```python
from build123d import *

# Parameters (mm, degrees)
SKETCH_1_R          = 1.6
SKETCH_1_R_2        = 29
SKETCH_1_R_3        = 1.1
EXTRUDE_1_DEPTH     = 2
FILLET_1_R          = 15
FILLET_2_R          = 10
FILLET_3_R          = 2
SKETCH_2_R          = 1.6
CUT_EXTRUDE_1_DEPTH = 124.188027016
CUT_EXTRUDE_2_DEPTH = 124.188027016
CUT_EXTRUDE_3_DEPTH = 124.188027016
FILLET_4_R          = 10


with BuildPart() as part:
    # 草图1 → 凸台-拉伸1 (new body)
    with BuildSketch(Plane.XY):
        with BuildLine():
            Line((0, 34), (0, 60))
            Line((0, 60), (-75, 60))
            Line((-75, 60), (-104.5, 42))
            Line((-104.5, 42), (-104.5, 10))
            Line((-104.5, 10), (-91.5, 10))
            Line((-91.5, 10), (-91.5, 0))
            Line((-91.5, 0), (-73.5, 0))
            Line((-73.5, 0), (-73.5, 6))
            Line((-73.5, 6), (-60.5, 6))
            Line((-60.5, 6), (-60.5, 0))
            Line((-60.5, 0), (-33, 0))
            Line((-33, 0), (-33, 6))
            Line((-33, 6), (-20, 6))
            Line((-20, 6), (-20, 0))
            Line((-20, 0), (0, 0))
            Line((0, 0), (5, 0))
            Line((5, 0), (8.183105221, -31.876446495))
            ThreePointArc((8.183105221, -31.876446495), (46.840501722, -65.154195343), (82, -28.2))
            Line((82, -28.2), (82, -2))
            Line((82, -2), (50, 34))
            Line((50, 34), (0, 34))
        make_face()
        with Locations((-86.5, 5)):
            Circle(SKETCH_1_R, mode=Mode.SUBTRACT)
        with Locations((-5, 5)):
            Circle(SKETCH_1_R, mode=Mode.SUBTRACT)
        with Locations((45, -28.2)):
            Circle(SKETCH_1_R_2, mode=Mode.SUBTRACT)
        with Locations((-35, 57)):
            Circle(SKETCH_1_R, mode=Mode.SUBTRACT)
        with Locations((-55, 57)):
            Circle(SKETCH_1_R, mode=Mode.SUBTRACT)
        with Locations((-87.5, 46.515606374)):
            Circle(SKETCH_1_R, mode=Mode.SUBTRACT)
        with Locations((-15.4, 48.1)):
            Circle(SKETCH_1_R_3, mode=Mode.SUBTRACT)
        with Locations((-15.4, 30.1)):
            Circle(SKETCH_1_R_3, mode=Mode.SUBTRACT)
        with Locations((-60.6, 48.1)):
            Circle(SKETCH_1_R_3, mode=Mode.SUBTRACT)
        with Locations((-60.6, 30.1)):
            Circle(SKETCH_1_R_3, mode=Mode.SUBTRACT)
        with Locations((-5, 55)):
            Circle(SKETCH_1_R, mode=Mode.SUBTRACT)
    extrude(amount=EXTRUDE_1_DEPTH)

    # 圆角1
    fillet_1_edges = [part.edges().sort_by_distance(p)[0] for p in [
        (0, 34, 1),
    ]]
    fillet(fillet_1_edges, radius=FILLET_1_R)

    # 圆角2
    fillet_2_edges = [part.edges().sort_by_distance(p)[0] for p in [
        (50, 34, 1),
        (82, -2, 1),
    ]]
    fillet(fillet_2_edges, radius=FILLET_2_R)

    # 圆角3
    fillet_3_edges = [part.edges().sort_by_distance(p)[0] for p in [
        (-20, 0, 1),
        (-20, 6, 1),
        (-33, 6, 1),
        (-33, 0, 1),
        (-60.5, 0, 1),
        (-60.5, 6, 1),
        (-73.5, 6, 1),
        (-73.5, 0, 1),
        (-91.5, 0, 1),
        (-91.5, 10, 1),
        (-104.5, 10, 1),
        (-104.5, 42, 1),
        (-75, 60, 1),
        (0, 60, 1),
        (5, 0, 1),
    ]]
    fillet(fillet_3_edges, radius=FILLET_3_R)

    # 草图2 → 切除-拉伸1 (cut, through all)
    with BuildSketch(Plane.XY.offset(2)):
        with Locations((67.627416998, -50.827416998)):
            Circle(SKETCH_2_R)
        with Locations((22.372583002, -50.827416998)):
            Circle(SKETCH_2_R)
        with Locations((22.372583002, -5.572583002)):
            Circle(SKETCH_2_R)
        with Locations((67.627416998, -5.572583002)):
            Circle(SKETCH_2_R)
    extrude(amount=-CUT_EXTRUDE_1_DEPTH, mode=Mode.SUBTRACT)

    # 草图3 → 切除-拉伸2 (cut, through all)
    with BuildSketch(Plane(origin=(0, 0, 0), x_dir=(-1, 0, 0), z_dir=(0, 0, -1))):
        with BuildLine():
            Line((20, 45.1), (20, 33.1))
            ThreePointArc((20, 33.1), (20.292893219, 32.392893219), (21, 32.1))
            Line((21, 32.1), (55, 32.1))
            ThreePointArc((55, 32.1), (55.707106781, 32.392893219), (56, 33.1))
            Line((56, 33.1), (56, 45.1))
            ThreePointArc((56, 45.1), (55.707106781, 45.807106781), (55, 46.1))
            Line((55, 46.1), (21, 46.1))
            ThreePointArc((21, 46.1), (20.292893219, 45.807106781), (20, 45.1))
        make_face()
        with BuildLine():
            Line((71.5, 20), (16, 20))
            ThreePointArc((16, 20), (12, 16), (16, 12))
            Line((16, 12), (71.5, 12))
            ThreePointArc((71.5, 12), (75.5, 16), (71.5, 20))
        make_face()
        with BuildLine():
            Line((79.5, 50), (79.5, 29))
            ThreePointArc((79.5, 29), (75.5, 25), (71.5, 29))
            Line((71.5, 29), (71.5, 50))
            ThreePointArc((71.5, 50), (75.5, 54), (79.5, 50))
        make_face()
        with BuildLine():
            Line((97.5, 37), (97.5, 18))
            ThreePointArc((97.5, 18), (92.5, 13), (87.5, 18))
            Line((87.5, 18), (87.5, 37))
            ThreePointArc((87.5, 37), (92.5, 42), (97.5, 37))
        make_face()
        with BuildLine():
            Line((-45.509339357, 26), (-12.653151788, 26))
            ThreePointArc((-12.653151788, 26), (-11.170341336, 25.342115182), (-10.663049368, 23.801273162))
            Line((-10.663049368, 23.801273162), (-12.946853034, 0.930667166))
            ThreePointArc((-12.946853034, 0.930667166), (-14.276095182, -0.758266904), (-16.368529004, -0.267243806))
            ThreePointArc((-16.368529004, -0.267243806), (-34.394913551, 10.368538233), (-55.324907134, 10.444485929))
            ThreePointArc((-55.324907134, 10.444485929), (-57.543460735, 11.326878506), (-57.335971128, 13.705437903))
            Line((-57.335971128, 13.705437903), (-47.004157994, 25.328727678))
            ThreePointArc((-47.004157994, 25.328727678), (-46.32865146, 25.824480112), (-45.509339357, 26))
        make_face()
    extrude(amount=-CUT_EXTRUDE_2_DEPTH, mode=Mode.SUBTRACT)

    # 草图4 → 切除-拉伸3 (cut, through all)
    with BuildSketch(Plane.XY.offset(2)):
        Polygon((67.777777778, 14), (82, -20.2), (96.250689627, 10.566455123), align=None)
    extrude(amount=-CUT_EXTRUDE_3_DEPTH, mode=Mode.SUBTRACT)

    # 圆角4
    fillet_4_edges = [part.edges().sort_by_distance(p)[0] for p in [
        (67.777777778, 14, 1),
        (82, -20.2, 1),
    ]]
    fillet(fillet_4_edges, radius=FILLET_4_R)


solid = part.part
```
Design review of the part built by this model. Coordinates are the model's own, in mm. A direction names the side the tool comes from. Coordinates: 2 decimals unless noted, no trailing zeros. Loops run counter-clockwise (first coordinate to the right, second up) from the corner with the lowest first, then second, coordinate; pieces in that order, holes last.
Q1. To check wall thickness, follow line 1 (Y direction, x = -53, z = 1.25); line 2 (X direction, y = 4, z = 1.6); line 3 (X direction, y = 27, z = 0.9). State the ranges of each line that lie inside material, in increasing order.
Reported:
line 1: y = 0 to 12, 20 to 32.1, 46.1 to 60
line 2: x = -91.5 to -87.75, -85.25 to -73.5, -60.5 to -33, -20 to -6.25, -3.75 to 12.64, 21.27 to 71.94
line 3: x = -104.5 to -97.5, -87.5 to -78.96, -72.04 to 56.22
Q2. Tool access review of faces 1 (the face through (-12, 16, 1)), 2 (the face through (-11.7, 16.2, 0)): name each direction out of +Z, -Z, +X, -X, +Y, -Y from which nothing blocks a thin tool from reaching the whole face with its end or side.
Reported:
face 1: +Z, -Z
face 2: -Z, +X, -X, +Y, -Y
Q3. We need section C-C on z = 0.4. State how many separate pieces and enclosed holes the cut face has, and give its area (3 significant figures).
Reported:
separate pieces: 1
enclosed holes: 20
area: 7,150 mm2
Q4. The part is to be moulded in two halves that separate along X. For faces 3 (the face through (74.74, -2.74, 1.01)), 4 (the face through (-11.7, 16.2, 2)), 5 (the face through (-75.4, 54, 1)), say which applies: +X half, -X half, draft (parallel to the pull), parting line (faces both ways), or undercut.
Reported:
face 3: +X half
face 4: draft
face 5: undercut
Q5. For pin 1 (0.6 mm diameter, centred on y = 53.5, z = 1, fed in from +X); pin 2 (1 mm diameter, centred on y = 39, z = 1, fed in from +X); pin 3 (3 mm diameter, centred on x = 67.63, y = -50.83, fed in from +Z); pin 4 (0.6 mm diameter, centred on x = -39.5, z = 1, fed in from -Y), all flat-tipped, find the tip position at first contact; note any pin that passes through.
Reported:
pin 1: stops at x = 0
pin 2: stops at x = 4.29
pin 3: passes through
pin 4: stops at y = 0
Q6. We need section B-B on y = -15. State the section outline as (x, z) points.
Reported:
outline: (6.5, 0) - (19.18, 0) - (19.18, 2) - (6.5, 2) - close; (70.82, 0) - (79.84, 0) - (79.84, 2) - (70.82, 2) - close
Q7. We need section A-A on x = -40.5. State the section outline as (y, z) points, and give its area (3 significant figures).
Reported:
outline: (0, 0) - (12, 0) - (12, 2) - (0, 2) - close; (20, 0) - (32.1, 0) - (32.1, 2) - (20, 2) - close; (46.1, 0) - (60, 0) - (60, 2) - (46.1, 2) - close
area: 76.0 mm2
